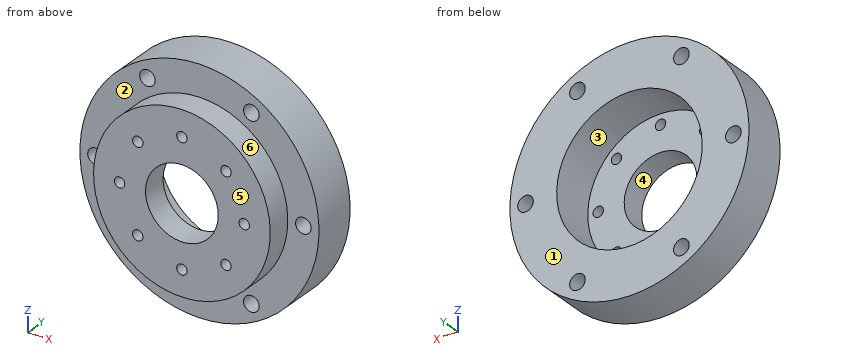
from build123d import *

# Parameters (mm, degrees)
SKETCH_1_R      = 17
SKETCH_1_R_2    = 1
SKETCH_1_R_3    = 7
EXTRUDE_1_DEPTH = 4.9
SKETCH_2_R      = 23
SKETCH_2_R_2    = 1.5
SKETCH_2_R_3    = 17
SKETCH_2_R_4    = 14
EXTRUDE_2_DEPTH = 6
SKETCH_3_R      = 23
SKETCH_3_R_2    = 14
SKETCH_3_R_3    = 1.5
EXTRUDE_3_DEPTH = 2.7


with BuildPart() as part:
    # 草图1 → 凸台-拉伸1 (new body)
    with BuildSketch(Plane(origin=(0, 0, 0), x_dir=(1, 0, 0), z_dir=(0, 1, 0))):
        with Locations(Location((0, 0, 0), (0, 0, 270))):
            Circle(SKETCH_1_R)
        with Locations(Location((8.485281374, -8.485281374, 0), (0, 0, 270))):
            Circle(SKETCH_1_R_2, mode=Mode.SUBTRACT)
        with Locations(Location((8.485281374, 8.485281374, 0), (0, 0, 270))):
            Circle(SKETCH_1_R_2, mode=Mode.SUBTRACT)
        with Locations(Location((0, -12, 0), (0, 0, 270))):
            Circle(SKETCH_1_R_2, mode=Mode.SUBTRACT)
        with Locations(Location((12, 0, 0), (0, 0, 270))):
            Circle(SKETCH_1_R_2, mode=Mode.SUBTRACT)
        with Locations(Location((0, 12, 0), (0, 0, 270))):
            Circle(SKETCH_1_R_2, mode=Mode.SUBTRACT)
        with Locations(Location((0, 0, 0), (0, 0, 270))):
            Circle(SKETCH_1_R_3, mode=Mode.SUBTRACT)
        with Locations(Location((-12, 0, 0), (0, 0, 270))):
            Circle(SKETCH_1_R_2, mode=Mode.SUBTRACT)
        with Locations(Location((-8.485281374, -8.485281374, 0), (0, 0, 270))):
            Circle(SKETCH_1_R_2, mode=Mode.SUBTRACT)
        with Locations(Location((-8.485281374, 8.485281374, 0), (0, 0, 270))):
            Circle(SKETCH_1_R_2, mode=Mode.SUBTRACT)
    extrude(amount=EXTRUDE_1_DEPTH)

    # 草图2 → 凸台-拉伸2 (add)
    # profile 1 of 2: a face of its own
    with BuildSketch(Plane(origin=(0, 4.9, 0), x_dir=(1, 0, 0), z_dir=(0, 1, 0))):
        with Locations(Location((0, 0, 0), (0, 0, 270))):
            Circle(SKETCH_2_R)
        with Locations(Location((-10, -17.320508076, 0), (0, 0, 270))):
            Circle(SKETCH_2_R_2, mode=Mode.SUBTRACT)
        with Locations(Location((-10, 17.320508076, 0), (0, 0, 270))):
            Circle(SKETCH_2_R_2, mode=Mode.SUBTRACT)
        with Locations(Location((10, 17.320508076, 0), (0, 0, 270))):
            Circle(SKETCH_2_R_2, mode=Mode.SUBTRACT)
        with Locations(Location((20, 0, 0), (0, 0, 270))):
            Circle(SKETCH_2_R_2, mode=Mode.SUBTRACT)
        with Locations(Location((-20, 0, 0), (0, 0, 270))):
            Circle(SKETCH_2_R_2, mode=Mode.SUBTRACT)
        with Locations(Location((10, -17.320508076, 0), (0, 0, 270))):
            Circle(SKETCH_2_R_2, mode=Mode.SUBTRACT)
        with Locations(Location((0, 0, 0), (0, 0, 270))):
            Circle(SKETCH_2_R_3, mode=Mode.SUBTRACT)
    # profile 2 of 2: a face of its own
    with BuildSketch(Plane(origin=(0, 4.9, 0), x_dir=(1, 0, 0), z_dir=(0, 1, 0))):
        with Locations(Location((0, 0, 0), (0, 0, 270))):
            Circle(SKETCH_2_R_3)
        with Locations(Location((0, 0, 0), (0, 0, 270))):
            Circle(SKETCH_2_R_4, mode=Mode.SUBTRACT)
    extrude(amount=EXTRUDE_2_DEPTH)

    # 草图3 → 凸台-拉伸3 (add)
    with BuildSketch(Plane(origin=(0, 10.9, 0), x_dir=(1, 0, 0), z_dir=(0, 1, 0))):
        with Locations(Location((0, 0, 0), (0, 0, 270))):
            Circle(SKETCH_3_R)
        with Locations(Location((0, 0, 0), (0, 0, 270))):
            Circle(SKETCH_3_R_2, mode=Mode.SUBTRACT)
        with Locations(Location((10, -17.320508076, 0), (0, 0, 270))):
            Circle(SKETCH_3_R_3, mode=Mode.SUBTRACT)
        with Locations(Location((20, 0, 0), (0, 0, 270))):
            Circle(SKETCH_3_R_3, mode=Mode.SUBTRACT)
        with Locations(Location((10, 17.320508076, 0), (0, 0, 270))):
            Circle(SKETCH_3_R_3, mode=Mode.SUBTRACT)
        with Locations(Location((-10, -17.320508076, 0), (0, 0, 270))):
            Circle(SKETCH_3_R_3, mode=Mode.SUBTRACT)
        with Locations(Location((-20, 0, 0), (0, 0, 270))):
            Circle(SKETCH_3_R_3, mode=Mode.SUBTRACT)
        with Locations(Location((-10, 17.320508076, 0), (0, 0, 270))):
            Circle(SKETCH_3_R_3, mode=Mode.SUBTRACT)
    extrude(amount=EXTRUDE_3_DEPTH)


solid = part.part
Geometry check sheet. Reference: the model listing, model coordinates, mm. Face numbers are marked on the shaded views. A direction names the side the tool comes from. Give positions to 0.01 mm unless a question says otherwise; leave off trailing zeros. Loops run counter-clockwise (first coordinate to the right, second up) from the corner with the lowest first, then second, coordinate; pieces in that order, holes last. Notation, with made-up numbers: M 67.25,39.5 L 122.25,39.5 A23 ccw 122.25,66.5 Z; hole C -35.5,17.5 d11. An arc over 180 degrees is marked long. Answer as a JSON object with one key per item and string values. Group by question number.
Item 1: Sectioned sample at A-A on x = 0. Record the boundary of the cut face in (y, z), plus the area to 3 significant figures.
Item 2: Sectioned sample at B-B on z = 0. Give the number of separate pieces and of enclosed holes in the cut face, plus the area to 3 significant figures.
Item 3: Material ranges on L1, parallel to X at y = 2.4, z = 0; L2, parallel to Z at x = 9, y = 3.5; L3, parallel to X at y = 7, z = 0, recorded low to high.
Item 4: Sectioned sample at D-D on z = 12. Record the boundary of the cut face in (x, y), plus the area to 3 significant figures.
Item 5: Mould release check, pull along Z, two halves, no side actions. Record for the marked faces 4, 5 and 6: pulls with the +Z half, pulls with the -Z half, needs draft (parallel to the pull), parting line crosses it, or undercut.
Item 6: Access from +Z, -Z, +X, -X, +Y, -Y to the whole of each face (thin tool, end or side, straight path). Record for the marked faces 1, 2 and 3.
Item 7: Gauge pin test, flat ends, axial feed: pin 1 (1.6 mm diameter, centred on x = 12, z = 0, fed in from -Y); pin 2 (4 mm diameter, centred on x = 17.5, y = 10.5, fed in from +Z); pin 3 (6 mm diameter, centred on y = 6.5, z = 2.5, fed in from +X); pin 4 (2 mm diameter, centred on y = 8.5, z = 12.5, fed in from -X). Record the tip position at first contact, or that the pin passes through.
Item 8: Sectioned sample at C-C on y = 10.75. Record the boundary of the cut face in (x, z).
Findings below:
{
 "1": {"outline": "M 0,-17 L 4.9,-17 L 4.9,-23 L 13.6,-23 L 13.6,-14 L 4.9,-14 L 4.9,-13 L 0,-13 Z; M 0,-11 L 4.9,-11 L 4.9,-7 L 0,-7 Z; M 0,7 L 4.9,7 L 4.9,11 L 0,11 Z; M 0,13 L 4.9,13 L 4.9,14 L 13.6,14 L 13.6,23 L 4.9,23 L 4.9,17 L 0,17 Z", "area": "235 mm2"},
 "2": {"separate pieces": "6", "enclosed holes": "0", "area": "183 mm2"},
 "3": {"L1": "-17 to -13, -11 to -7, 7 to 11, 13 to 17", "L2": "-14.42 to -9.34, -7.63 to 7.63, 9.34 to 14.42", "L3": "-23 to -21.5, -18.5 to -14, 14 to 18.5, 21.5 to 23"},
 "4": {"outline": "M -19.62,4.9 L -12.04,4.9 L -12.04,0 L -1,0 L -1,4.9 L -7.21,4.9 L -7.21,13.6 L -19.62,13.6 Z; M 1,0 L 12.04,0 L 12.04,4.9 L 19.62,4.9 L 19.62,13.6 L 7.21,13.6 L 7.21,4.9 L 1,4.9 Z", "area": "324 mm2"},
 "5": {"face 4": "undercut", "face 5": "needs draft", "face 6": "parting line crosses it"},
 "6": {"face 1": "+Z, -Z, +X, -X, +Y", "face 2": "-Y", "face 3": "+Y"},
 "7": {"pin 1": "through", "pin 2": "z = 16.99", "pin 3": "x = 23", "pin 4": "x = -19.92"},
 "8": {"outline": "C 0,0 d46; hole C -20,0 d3; hole C 0,0 d28; hole C -10,-17.32 d3; hole C -10,17.32 d3; hole C 10,-17.32 d3; hole C 10,17.32 d3; hole C 20,0 d3"}
}
